```python
from build123d import *

# Parameters (mm, degrees)
F0_R            = 22.5
F0_R_2          = 4.515
F0_R_3          = 5
F1_DEPTH        = 17.5
F2_R            = 4.825
F3_DEPTH        = 19.15
F3_COPIES_COUNT = 6


# Not quite as in the source:
# - a pattern or mirror of a feature is missing from the dataset's text; its kind, count and spacing are read off the source's solid


with BuildPart() as f1:
    # F0 (on Front) → F1 (new body, symmetric)
    with BuildSketch(Plane.XZ):
        Circle(F0_R)
        with Locations((-12.9903810568, -7.5)):
            Circle(F0_R_2, mode=Mode.SUBTRACT)
        with Locations((0, -15)):
            Circle(F0_R_2, mode=Mode.SUBTRACT)
        with Locations((12.9903810568, -7.5)):
            Circle(F0_R_2, mode=Mode.SUBTRACT)
        with Locations((-12.9903810568, 7.5)):
            Circle(F0_R_2, mode=Mode.SUBTRACT)
        Circle(F0_R_3, mode=Mode.SUBTRACT)
        with Locations((12.9903810568, 7.5)):
            Circle(F0_R_2, mode=Mode.SUBTRACT)
        with Locations((0, 15)):
            Circle(F0_R_2, mode=Mode.SUBTRACT)
    extrude(amount=F1_DEPTH, both=True)

    # F2 (on face) → F3 (cut)
    with BuildSketch(Plane(origin=(0, 17.5, 0), x_dir=(-1, 0, 0), z_dir=(0, 1, 0))):
        with Locations((0, 15)):
            Circle(F2_R)
    f3 = extrude(amount=-F3_DEPTH, mode=Mode.SUBTRACT)

    # F3_copies: F3 ×6 about axis
    f3_copies_axis = Axis((0, 0, 0), (0, 1, 0))
    for i in range(1, F3_COPIES_COUNT):
        add(f3.rotate(f3_copies_axis, i * 360 / F3_COPIES_COUNT), mode=Mode.SUBTRACT)


solid = f1.part
```
Check sheet for the modelled part. Datum: model origin and axes. Units: mm. A direction names the side the tool comes from. Give positions to 0.01 mm unless a question says otherwise; leave off trailing zeros. Loops run counter-clockwise (first coordinate to the right, second up) from the corner with the lowest first, then second, coordinate; pieces in that order, holes last. Notation, with made-up numbers: M 48,45.25 L 54,45.25 A18 cw 54,61.25 Z; hole C 38,24.5 d2. An arc over 180 degrees is marked long. Answer in a Markdown table with one row per item.
1) Tool access check on faces 4 (the face through (0.628, 8.059, 19.784)), 5 (the face through (17.297, -9.464, -6.144)). Record the directions out of +Z, -Z, +X, -X, +Y, -Y that give a thin tool (end or side, any length) a straight path to the whole face; none if there is none.
Solutions:
| item | result |
|---|---|
| face 4 | +Y |
| face 5 | +Y, -Y |
2) Thickness scan on line 1 (Z direction, x = 0, y = 13) (3 decimals); line 2 (Z direction, x = -16.5, y = -12); line 3 (Z direction, x = 15.5, y = 0). Record the ranges inside material, lowest first.
Solutions:
| item | result |
|---|---|
| line 1 | z = -22.5 to -19.825, -10.175 to -5, 5 to 10.175, 19.825 to 22.5 |
| line 2 | z = -15.3 to -10.34, -4.66 to 4.66, 10.34 to 15.3 |
| line 3 | z = -16.31 to -11.62, -3.38 to 3.38, 11.62 to 16.31 |
3) Cross-section at C-C (y = -15). Enter the section's corners in (x, z) (3 decimals), plus the area to 3 significant figures.
Solutions:
| item | result |
|---|---|
| outline | C 0,0 d45; hole C -12.99,-7.5 d9.03; hole C -12.99,7.5 d9.03; hole C 0,0 d10; hole C 0,-15 d9.03; hole C 0,15 d9.03; hole C 12.99,-7.5 d9.03; hole C 12.99,7.5 d9.03 |
| area | 1,130 mm^2 |
4) Cross-section at D-D (z = -7.5). Enter the section's corners in (x, y), plus the area to 3 significant figures.
Solutions:
| item | result |
|---|---|
| outline | M -21.21,-17.5 L -17.51,-17.5 L -17.51,-1.65 L -17.82,-1.65 L -17.82,17.5 L -21.21,17.5 Z; M -8.48,-17.5 L 8.48,-17.5 L 8.48,-1.65 L 8.17,-1.65 L 8.17,17.5 L -8.17,17.5 L -8.17,-1.65 L -8.48,-1.65 Z; M 17.51,-17.5 L 21.21,-17.5 L 21.21,17.5 L 17.82,17.5 L 17.82,-1.65 L 17.51,-1.65 Z |
| area | 829 mm^2 |
5) Depth check by flat-ended pin: pin 1 (5 mm diameter, centred on x = -6, y = -8, fed in from -Z); pin 2 (2 mm diameter, centred on y = -7.5, z = -11.5, fed in from -X); pin 3 (1 mm diameter, centred on x = 17.5, y = 7, fed in from +Z). Enter the tip coordinate at first touch or a pass-through.
Solutions:
| item | result |
|---|---|
| pin 1 | stops at z = -22.23 |
| pin 2 | stops at x = -19.9 |
| pin 3 | stops at z = 14.74 |
6) Mould release check, pull along Z, two halves, no side actions. Record for faces 1 (the face through (-0.3, 17.5, 5.3)), 2 (the face through (10.382, -0.245, -19.961)), 3 (the face through (-10.563, -9.464, 11.307)): released by +Z, released by -Z, zero draft, split by the parting line, or undercut.
Solutions:
| item | result |
|---|---|
| face 1 | zero draft |
| face 2 | split by the parting line |
| face 3 | undercut |
7) Cross-section at A-A (z = 0). Enter the section's corners in (x, y), plus the area to 4 significant figures.
Solutions:
| item | result |
|---|---|
| outline | M -22.5,-17.5 L -5,-17.5 L -5,17.5 L -22.5,17.5 Z; M 5,-17.5 L 22.5,-17.5 L 22.5,17.5 L 5,17.5 Z |
| area | 1,225 mm^2 |
8) Cross-section at B-B (x = 0). Enter the section's corners in (y, z) (3 decimals), plus the area to 3 significant figures.
Solutions:
| item | result |
|---|---|
| outline | M -17.5,-22.5 L 17.5,-22.5 L 17.5,-19.825 L -1.65,-19.825 L -1.65,-19.515 L -17.5,-19.515 Z; M -17.5,-10.485 L -1.65,-10.485 L -1.65,-10.175 L 17.5,-10.175 L 17.5,-5 L -17.5,-5 Z; M -17.5,5 L 17.5,5 L 17.5,10.175 L -1.65,10.175 L -1.65,10.485 L -17.5,10.485 Z; M -17.5,19.515 L -1.65,19.515 L -1.65,19.825 L 17.5,19.825 L 17.5,22.5 L -17.5,22.5 Z |
| area | 569 mm^2 |
